Build history of the part. All positions in model axes, mm. Round coordinates to 2 decimals unless told otherwise and drop trailing zeros. Loops run counter-clockwise (first coordinate to the right, second up) from the corner with the lowest first, then second, coordinate; pieces in that order, holes last. Notation, with made-up numbers: (0, 15) - (10, 15) arc R27 cw to (10, 34) - close; hole circle Ø9 at (-2, 58). An arc over 180 degrees is marked (long way). Use a Markdown table: item, result.
from build123d import *

# Parameters (mm, degrees)
SKETCH1_R               = 4.5
BOSS_EXTRUDE1_DEPTH     = 0.8
SKETCH2_R               = 0.767914883
SKETCH2_R_2             = 0.3556
SKETCH2_R_3             = 4.5
CUT_EXTRUDE1_DEPTH      = 27.149953829
CUT_EXTRUDE2_DEPTH      = 27.149953829
CUT_EXTRUDE2_DEPTH_BACK = 27.149953829
SKETCH3_R               = 0.889


with BuildPart() as part:
    # Sketch1 → Boss-Extrude1 (new body)
    with BuildSketch(Plane(origin=(0, 0, -38.7925), x_dir=(-1, 0, 0), z_dir=(0, 0, -1))):
        with BuildLine():
            Line((23.8125, 6.6675), (-23.8125, 6.6675))
            ThreePointArc((-23.8125, 6.6675), (-25.272010309, 5.153242143), (-23.705057143, 3.750457422))
            ThreePointArc((-23.705057143, 3.750457422), (-23.130382387, 3.548805041), (-22.887, 2.990522163))
            Line((-22.887, 2.990522163), (-22.887, -2.990522163))
            ThreePointArc((-22.887, -2.990522163), (-23.130382387, -3.548805041), (-23.705057143, -3.750457422))
            ThreePointArc((-23.705057143, -3.750457422), (-25.272010309, -5.153242143), (-23.8125, -6.6675))
            Line((-23.8125, -6.6675), (23.8125, -6.6675))
            ThreePointArc((23.8125, -6.6675), (25.272010309, -5.153242143), (23.705057143, -3.750457422))
            ThreePointArc((23.705057143, -3.750457422), (23.130382387, -3.548805041), (22.887, -2.990522163))
            Line((22.887, -2.990522163), (22.887, 2.990522163))
            ThreePointArc((22.887, 2.990522163), (23.130382387, 3.548805041), (23.705057143, 3.750457422))
            ThreePointArc((23.705057143, 3.750457422), (25.272010309, 5.153242143), (23.8125, 6.6675))
        make_face()
        with Locations((16.51, 0)):
            Circle(SKETCH1_R, mode=Mode.SUBTRACT)
        Circle(SKETCH1_R, mode=Mode.SUBTRACT)
        with Locations((-16.51, 0)):
            Circle(SKETCH1_R, mode=Mode.SUBTRACT)
    extrude(amount=BOSS_EXTRUDE1_DEPTH)

    # Sketch2 → Cut-Extrude1 (cut, through all)
    with BuildSketch(Plane(origin=(0, 0, -39.5925), x_dir=(-1, 0, 0), z_dir=(0, 0, -1))):
        with Locations((-12.077914883, -4.432085117)):
            Circle(SKETCH2_R)
        with Locations((-20.942085117, 4.432085117)):
            Circle(SKETCH2_R)
        with Locations((-4.432085117, 4.432085117)):
            Circle(SKETCH2_R)
        with Locations((-7.62, -1.905)):
            Circle(SKETCH2_R_2)
        with Locations((20.942085117, -4.432085117)):
            Circle(SKETCH2_R)
        with Locations((12.077914883, 4.432085117)):
            Circle(SKETCH2_R)
        with Locations((4.432085117, -4.432085117)):
            Circle(SKETCH2_R)
        with Locations((-8.89, -1.905)):
            Circle(SKETCH2_R_2)
        with Locations((-7.62, 1.905)):
            Circle(SKETCH2_R_2)
        with Locations((-8.89, 1.905)):
            Circle(SKETCH2_R_2)
        with Locations((-7.62, 0.635)):
            Circle(SKETCH2_R_2)
        with Locations((-8.89, 0.635)):
            Circle(SKETCH2_R_2)
        Circle(SKETCH2_R_3)
        with Locations((-7.62, -0.635)):
            Circle(SKETCH2_R_2)
        with Locations((-8.89, -0.635)):
            Circle(SKETCH2_R_2)
        with Locations((8.89, 1.905)):
            Circle(SKETCH2_R_2)
        with Locations((7.62, 1.905)):
            Circle(SKETCH2_R_2)
        with Locations((8.89, -1.905)):
            Circle(SKETCH2_R_2)
        with Locations((7.62, -1.905)):
            Circle(SKETCH2_R_2)
        with Locations((8.89, -0.635)):
            Circle(SKETCH2_R_2)
        with Locations((7.62, -0.635)):
            Circle(SKETCH2_R_2)
        with Locations((8.89, 0.635)):
            Circle(SKETCH2_R_2)
        with Locations((7.62, 0.635)):
            Circle(SKETCH2_R_2)
    extrude(amount=-CUT_EXTRUDE1_DEPTH, mode=Mode.SUBTRACT)

    # Sketch3 → Cut-Extrude2 (cut, two sides: drawn at the far end of the back side and taken through both)
    with BuildSketch(Plane(origin=(0, 0, -39.5925), x_dir=(-1, 0, 0), z_dir=(0, 0, -1)).offset(-CUT_EXTRUDE2_DEPTH_BACK)):
        with Locations((-23.8125, 5.207)):
            Circle(SKETCH3_R)
        with Locations((-23.8125, -5.207)):
            Circle(SKETCH3_R)
        with Locations((23.8125, 5.207)):
            Circle(SKETCH3_R)
        with Locations((23.8125, -5.207)):
            Circle(SKETCH3_R)
        with Locations((-8.255, 4.953)):
            Circle(SKETCH3_R)
        with Locations((8.255, 4.953)):
            Circle(SKETCH3_R)
        with Locations((8.255, -4.953)):
            Circle(SKETCH3_R)
        with Locations((-8.255, -4.953)):
            Circle(SKETCH3_R)
    extrude(amount=CUT_EXTRUDE2_DEPTH + CUT_EXTRUDE2_DEPTH_BACK, mode=Mode.SUBTRACT)


solid = part.part
Q1. Cut at A-A, the plane x = 0. List the corners of the cut face in (y, z), plus the area to 3 significant figures.
Results found:
| item | result |
|---|---|
| outline | (-6.67, -39.59) - (-4.5, -39.59) - (-4.5, -38.79) - (-6.67, -38.79) - close; (4.5, -39.59) - (6.67, -39.59) - (6.67, -38.79) - (4.5, -38.79) - close |
| area | 3.47 mm2 |
Q2. Cut at C-C, the plane z = -39.15. Count the separate pieces of the cut face and the enclosed holes in it, plus the area to 3 significant figures.
Results found:
| item | result |
|---|---|
| separate pieces | 1 |
| enclosed holes | 33 |
| area | 407 mm2 |
Q3. Probe line 1 (X direction, y = 5.75, z = -39); line 2 (X direction, y = -2.5, z = -39.45); line 3 (Y direction, x = -20.5, z = -39.5). List the from-to ranges inside material, lowest first.
Results found:
| item | result |
|---|---|
| line 1 | x = -25.17 to -24.52, -23.11 to -8.65, -7.86 to 7.86, 8.65 to 23.11, 24.52 to 25.17 |
| line 2 | x = -22.89 to -20.25, -12.77 to -3.74, 3.74 to 12.77, 20.25 to 22.89 |
| line 3 | y = -6.67 to -5.06, -3.8 to -2.08, 2.08 to 6.67 |
Q4. Pull direction Y, two halves, no side cores. Call faces 1 (the face through (-25.27, 5.12, -39.19)), 2 (the face through (0, 5, -38.792)): pulls with the +Y half, pulls with the -Y half, needs draft (parallel to the pull), parting line crosses it, or undercut.
Results found:
| item | result |
|---|---|
| face 1 | undercut |
| face 2 | needs draft |
Q5. Cut at B-B, the plane x = -14. List the corners of the cut face in (y, z), plus the area to 3 significant figures.
Results found:
| item | result |
|---|---|
| outline | (-6.67, -39.59) - (-3.73, -39.59) - (-3.73, -38.79) - (-6.67, -38.79) - close; (3.73, -39.59) - (6.67, -39.59) - (6.67, -38.79) - (3.73, -38.79) - close |
| area | 4.69 mm2 |
